Can you work these out from the model? Positions are in its coordinate system, mm. Face numbers are marked on the shaded views. A direction names the side the tool comes from. Give positions to 0.01 mm unless a question says otherwise; leave off trailing zeros. Loops run counter-clockwise (first coordinate to the right, second up) from the corner with the lowest first, then second, coordinate; pieces in that order, holes last. Notation, with made-up numbers: M 43.25,-39.75 L 87.25,-39.75 A25 ccw 87.25,-2.75 Z; hole C -31.5,20 d10. An arc over 180 degrees is marked long. Use CSV: the item, a comma, the result in double quotes.
Autodesk Inventor part; units mm, degrees
ref_plane "Pracovní rovina1" through (0, 12.5, 0) normal (0, -1, 0) x (1, 0, 0)
ref_plane "YZ Plane" through (0, 0, 0) normal (1, 0, 0) x (0, 1, 0)
ref_plane "XZ Plane" through (0, 0, 0) normal (0, 1, 0) x (-1, 0, 0)
sketch "Náčrt1" plane through (0, 0, 0) normal (0, 0, 1) x (1, 0, 0)
  circle A0 centre (0, 0) radius 14
  dimension "d0" = 28
extrude "Vysunutí1" add sketch "Náčrt1" along normal mid plane 25
sketch "Náčrt2" plane through (0, 0, 0) normal (1, 0, 0) x (0, 1, 0)
  line L0 (-14, -12.5) -> (14, -12.5)
  line L1 (14, 12.5) -> (-14, 12.5)
  line L2 (14, -12.5) -> (14, 12.5)
  line L3 (14, 11) -> (12.5, 11)
  line L4 (12.5, 11) -> (12.5, -11)
  line L5 (12.5, -11) -> (14, -11)
  line L6 (14, -11) -> (14, 11)
  line L7 (14, 0) -> (-14, 0) construction
  line L8 (-14, -12.5) -> (-14, 12.5)
  line L9 (0, 12.5) -> (0, -12.5) construction
  point P0 (0, 0)
  point P1 (14, -11)
  dimension "d4" = 11
  dimension "d5" = 12.5
revolve "Rotace1" cut sketch "Náčrt2" angle 360 about axis through (0, 0, 12.5) along (0, 0, -1) contours L5 L4 L3 L2
sketch "Náčrt3" plane through (0, 0, -12.5) normal (0, 0, -1) x (-1, 0, 0)
  line L0 (-6, 5) -> (6, 5)
  line L1 (6, 5) -> (6, -5)
  line L2 (6, -5) -> (-6, -5)
  line L3 (-6, -5) -> (-6, 5)
  line L4 (-6, 5) -> (6, -5) construction
  line L5 (6, 5) -> (-6, -5) construction
  circle A0 centre (0, 0) radius 9
  dimension "d7" = 12
  dimension "d8" = 10
  dimension "d9" = 18
hole "Díra1" at (0, 0, -12.5) direction (0, 0, 1) diameter 18 depth 10
sketch "Náčrt4" plane through (0, 0, 12.5) normal (0, 0, 1) x (1, 0, 0)
  circle A0 centre (0, 0) radius 14
hole "Díra2" at (0, 0, 12.5) direction (0, 0, -1) diameter 3 end through all
ref_plane "Pracovní rovina1" through (0, 12.5, 0) normal (0, -1, 0) x (1, 0, 0)
sketch "Náčrt5" plane through (0, 12.5, 0) normal (0, -1, 0) x (1, 0, 0)
  line L0 (1.5, -2.5) -> (-1.5, -2.5)
  line L1 (-9, -2.5) -> (9, -2.5)
  line L2 (0, 0) -> (0, -10.7479) construction
  point P0 (0, 4.5)
  dimension "d24" = 2.5
  dimension "d25" = 4.5
hole "Díra3" at (0, 12.5, 0) at (0, 12.5, 4.5) direction (0, -1, 0) diameter 3 depth 12.5
thread "Závit1"
thread "Závit2"
chamfer "Zkosení1" distance 1 angle 45 1 edges at (0, -9, -12.5)
fillet "Zaoblení1" radius 1 1 edges at (0, -9, -2.5)
chamfer "Zkosení2" distance 0.5 angle 45 1 edges at (0, 1.5, -2.5)
properties part number "Wheel" material "Mosaz, měkká žlutá"
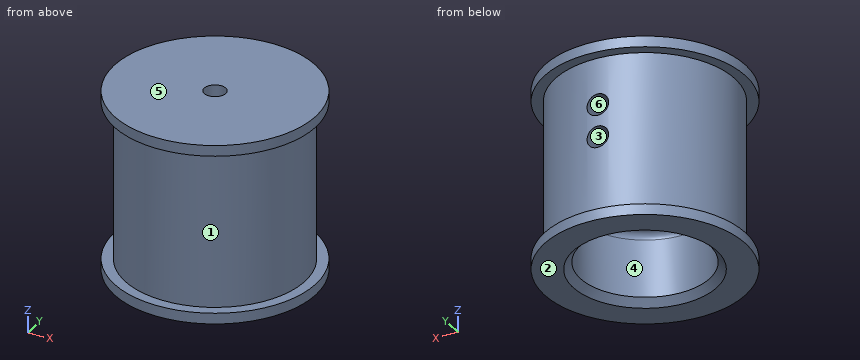
Q1. I want a section at D-D, the plane z = -9. Please give me the cut outline in (x, y), then the cut area to 3 significant figures.
Model answer:
outline,"C 0,0 d25; hole C 0,0 d18"
area,"236 mm2"
Q2. I want a section at C-C, the plane x = 12. Please give me the cut outline in (y, z), then the cut area to 3 significant figures.
Model answer:
outline,"M -7.21,-12.5 L 7.21,-12.5 L 7.21,-11 L 3.5,-11 L 3.5,11 L 7.21,11 L 7.21,12.5 L -7.21,12.5 L -7.21,11 L -3.5,11 L -3.5,-11 L -7.21,-11 Z"
area,"197 mm2"
Q3. For the marked faces 4, 5 and 6, which set-ups out of +Z, -Z, +X, -X, +Y, -Y let a thin tool reach every point of the face, with its end or its side?
Model answer:
face 4,"-Z"
face 5,"+Z, +X, -X, +Y, -Y"
face 6,"+Y"
Q4. I want a section at B-B, the plane z = 10. Please give me the cut outline in (x, y).
Model answer:
outline,"C 0,0 d25; hole C 0,0 d3"
Q5. I'm going to push flat-ended pins straight in: P1, Ø5, axis at y = -11, z = -5, coming from the +X side; P2, Ø4, axis at x = 0, z = 4.5, coming from the -Y side; P3, Ø1.5, axis at y = 5.5, z = 6, coming from the -X side; P4, Ø1.8, axis at x = 0, y = 0, coming from the +Z side. Where does each tip first touch, or does it pass through?
Model answer:
P1,"x = 9.17"
P2,"y = -12.5"
P3,"x = -11.56"
P4,"through"
Q6. I want a section at A-A, the plane x = 0. State how many separate pieces and enclosed holes the cut face has, then the cut area to 3 significant figures.
Model answer:
separate pieces,"4"
enclosed holes,"0"
area,"342 mm2"
Q7. If we mould it in two halves opening along X, with no side actions, what happens to the marked faces 1, 2 and 3? For each: released by +X, released by -X, zero draft, split by the parting line, or undercut.
Model answer:
face 1,"split by the parting line"
face 2,"zero draft"
face 3,"undercut"
Q8. Please list where these lines run through material, in increasing order: L1, parallel to Z at x = 0, y = 6; L2, parallel to X at y = 0, z = 8.5; L3, parallel to X at y = 0, z = -7. Write a range as from..to.
Model answer:
L1,"-2.5..-1.5, 1.5..3, 6..12.5"
L2,"-12.5..-1.5, 1.5..12.5"
L3,"-12.5..-9, 9..12.5"
